Check sheet for the modelled part. Datum: model origin and axes. Units: mm. Face numbers are marked on the shaded views. A direction names the side the tool comes from. Round coordinates to 2 decimals unless told otherwise and drop trailing zeros. Loops run counter-clockwise (first coordinate to the right, second up) from the corner with the lowest first, then second, coordinate; pieces in that order, holes last. Notation, with made-up numbers: (59, 40) - (83, 40) arc R35 ccw to (83, 74) - close; hole circle Ø9 at (43.25, 20). An arc over 180 degrees is marked (long way). Return JSON: item names as keys, results as strings.
from build123d import *

# Parameters (mm, degrees)
EXTRUDE_1_DEPTH = 5


with BuildPart() as part:
    # Эскиз1 → Бобышка-Вытянуть1 (new body)
    with BuildSketch(Plane.XY):
        with BuildLine():
            Line((-80, 11.347450151), (-76.287415542, 14.809491167))
            ThreePointArc((-76.287415542, 14.809491167), (-43.024892089, -14.449127714), (0, -25))
            Line((0, -25), (0, -12.6))
            ThreePointArc((0, -12.6), (-1.6, -11), (0, -9.4))
            Line((0, -9.4), (0, 0))
            ThreePointArc((0, 0), (-37.578310294, 4.533812859), (-73, 17.875055754))
            Line((-73, 17.875055754), (-70.492401879, 20.213428832))
            ThreePointArc((-70.492401879, 20.213428832), (-75.677514984, 24.687695279), (-80, 30))
            ThreePointArc((-80, 30), (-80.662257492, 20.673725075), (-80, 11.347450151))
        make_face()
    extrude(amount=EXTRUDE_1_DEPTH)


solid = part.part
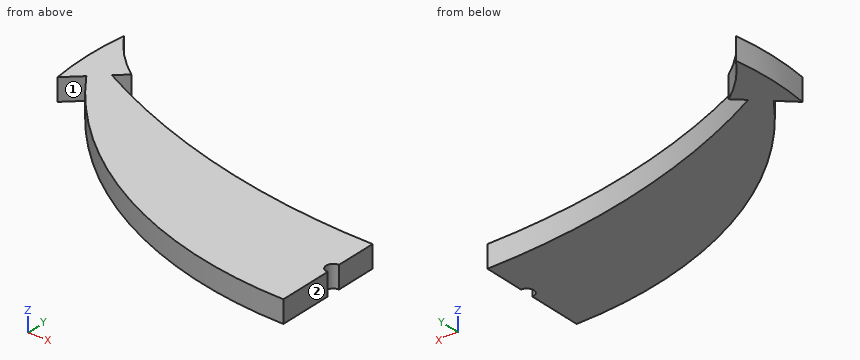
Q1. Depth check by flat-ended pin: P1, Ø2, axis at x = -15.5, z = 2.5, coming from the +Y side; P2, Ø1, axis at y = -19, z = 4, coming from the +X side. Enter the tip coordinate at first touch or a pass-through.
Answer key:
{"P1": "stops at y = 0.86", "P2": "stops at x = 0"}
Q2. Sectioned sample at B-B (x = -61.5). Enter the section's corners in (y, z), plus the area to 3 significant figures.
Answer key:
{"outline": "(-1.76, 0) - (12.46, 0) - (12.46, 5) - (-1.76, 5) - close", "area": "71.1 mm²"}
Q3. Sectioned sample at A-A (z = 3.75). Enter the section's corners in (x, y), plus the area to 3 significant figures.
Answer key:
{"outline": "(-80, 11.35) - (-76.29, 14.81) arc R93 ccw to (0, -25) - (0, -12.6) arc R1.6 cw to (0, -9.4) - (0, 0) arc R158 cw to (-73, 17.88) - (-70.49, 20.21) arc R39 cw to (-80, 30) arc R66 ccw to start", "area": "1,570 mm²"}
Q4. Scan lines: probe 1 along X at (y, z) = (13.5, 2.95); probe 2 along Y at (x, z) = (-71.5, 0.9); probe 3 along Y at (x, z) = (-25, 2.95). Record each from-to range of solid material in increasing order. Write a range as [from, to].
Answer key:
{"probe 1": "x = [-80.27, -77.69], [-75.36, -63.9]", "probe 2": "y = [8.53, 17.1], [19.27, 20.96]", "probe 3": "y = [-21.58, 1.99]"}
Q5. Tool access check on the marked faces 1 and 2. Record the directions out of +Z, -Z, +X, -X, +Y, -Y that give a thin tool (end or side, any length) a straight path to the whole face; none if there is none.
Answer key:
{"face 1": "+Z, -Z, -Y", "face 2": "+Z, -Z, +X, +Y, -Y"}
Q6. Sectioned sample at C-C (y = -11). Enter the section's corners in (x, z).
Answer key:
{"outline": "(-49.07, 0) - (-1.6, 0) - (-1.6, 5) - (-49.07, 5) - close"}
